Check sheet for the modelled part. Datum: model origin and axes. Units: mm. Round coordinates to 2 decimals unless told otherwise and drop trailing zeros. Loops run counter-clockwise (first coordinate to the right, second up) from the corner with the lowest first, then second, coordinate; pieces in that order, holes last. Notation, with made-up numbers: (66.25, -2.75) -> (101.25, -2.75) arc R10 cw to (101.25, 16.25) -> close; hole circle Ø11 at (60.5, -37). An arc over 180 degrees is marked (long way). One line per question, with ' | ' between items.
```python
from build123d import *

# Parameters (mm, degrees)
F0_R     = 9.779
F1_DEPTH = 6.35


with BuildPart() as f1:
    # F0 (on Top) → F1 (new body)
    with BuildSketch(Plane.XY):
        Circle(F0_R)
        with BuildLine():
            ThreePointArc((3.473407, -6.418978), (1.16965, -7.586652), (1.58991, -5.038292))
            ThreePointArc((1.58991, -5.038292), (2.881563, -5.251304), (3.473407, -6.418978))
        make_face(mode=Mode.SUBTRACT)
        with BuildLine():
            ThreePointArc((-5.124001, 1.455262), (-5.132588, 1.297819), (-5.158244, 1.142243))
            ThreePointArc((-5.158244, 1.142243), (-8.011015, 1.612705), (-5.124001, 1.455262))
        make_face(mode=Mode.SUBTRACT)
        with BuildLine():
            ThreePointArc((2.144431, 2.341375), (2.905959, 1.279073), (3.175, 0))
            ThreePointArc((3.175, 0), (2.560689, -1.877098), (0.955475, -3.02782))
            ThreePointArc((0.955475, -3.02782), (-2.144431, -2.341375), (-3.099906, 0.686444))
            ThreePointArc((-3.099906, 0.686444), (-0.955475, 3.02782), (2.144431, 2.341375))
        make_face(mode=Mode.SUBTRACT)
        with BuildLine():
            ThreePointArc((5.993995, 4.963716), (5.129452, 3.638599), (3.568334, 3.896049))
            ThreePointArc((3.568334, 3.896049), (3.962937, 6.288833), (5.993995, 4.963716))
        make_face(mode=Mode.SUBTRACT)
    extrude(amount=F1_DEPTH)


solid = f1.part
```
(1) Go/stop test with flat-tipped pins: pin 1 (10 mm diameter, centred on x = 5, y = 7.5, fed in from -Z); pin 2 (2 mm diameter, centred on y = -7.5, z = 2, fed in from +X). Record where each tip stops, or that it passes through.
Answer:
pin 1: stops at z = 0 | pin 2: stops at x = 7.31
(2) Sectioned sample at D-D, the plane y = 0.25. Record the cut outline in (x, z), and give its area (3 significant figures).
Answer:
outline: (-9.78, 0) -> (-7.37, 0) -> (-7.37, 6.35) -> (-9.78, 6.35) -> close; (-5.77, 0) -> (-3.17, 0) -> (-3.17, 6.35) -> (-5.77, 6.35) -> close; (3.17, 0) -> (9.78, 0) -> (9.78, 6.35) -> (3.17, 6.35) -> close | area: 73.8 mm2
(3) Sectioned sample at C-C, the plane z = 4.75. Record the cut outline in (x, y) (3 decimals), and give its area (3 significant figures).
Answer:
outline: circle Ø19.558 at (0, 0); hole (-5.158, 1.142) arc R1.448 ccw to (-5.124, 1.455) arc R1.448 ccw (long way) to start; hole (-3.1, 0.686) arc R3.175 ccw to (0.955, -3.028) arc R3.175 ccw to (3.175, 0) arc R3.175 ccw to (2.144, 2.341) arc R3.175 ccw to start; hole (1.59, -5.038) arc R1.448 ccw (long way) to (3.473, -6.419) arc R1.448 ccw to start; hole circle Ø2.896 at (4.546, 4.964) | area: 249 mm2
(4) Scan lines: probe 1 along Y at (x, z) = (2, 1.25); probe 2 along Y at (x, z) = (1.5, 2); probe 3 along X at (y, z) = (-1.25, 5.5). Record each from-to range of solid material in increasing order.
Answer:
probe 1: y = -9.57 to -7.87, -4.97 to -2.47, 2.47 to 9.57 | probe 2: y = -9.66 to -7.77, -5.07 to -2.8, 2.8 to 9.66 | probe 3: x = -9.7 to -2.92, 2.92 to 9.7
(5) Sectioned sample at A-A, the plane y = -5.5. Record the cut outline in (x, z).
Answer:
outline: (-8.09, 0) -> (0.91, 0) -> (0.91, 6.35) -> (-8.09, 6.35) -> close; (3.14, 0) -> (8.09, 0) -> (8.09, 6.35) -> (3.14, 6.35) -> close
(6) Sectioned sample at B-B, the plane x = 0. Record the cut outline in (y, z) (3 decimals).
Answer:
outline: (-9.779, 0) -> (-3.175, 0) -> (-3.175, 6.35) -> (-9.779, 6.35) -> close; (3.175, 0) -> (9.779, 0) -> (9.779, 6.35) -> (3.175, 6.35) -> close
(7) Mould release check, pull along Y, two halves, no side actions. Record for faces 1 (the face through (4, 0, 6.35)), 2 (the face through (-8.016, 1.551, 3.131)), 3 (the face through (-2.12, -9.546, 3.131)): +Y half, -Y half, draft (parallel to the pull), parting line (faces both ways), or undercut.
Answer:
face 1: draft | face 2: undercut | face 3: parting line
